Read the model definition and answer for the solid it produces. Units are mm, in the model's axes. A direction names the side the tool comes from. Coordinates: 2 decimals unless noted, no trailing zeros. Write each loop counter-clockwise with the first axis right and the second up, starting at its lowest first coordinate (ties: lowest second). Pieces come first, ordered by that corner, then holes.
(1) The mould has two halves that part along X. Classify faces 1 (the cylindrical face through (25.116, -3.788, 4.684)), 2 (the cylindrical face through (18.45, 9.9, 10.98)), 3 (the flat face through (-16, 9, 12.5)), 4 (the flat face through (-4.64, 5.73, 6.2)): +X half, -X half, draft (parallel to the pull), parting line (faces both ways), or undercut.
(2) Find the intervals of material crossed by probe 1 along X at (y, z) = (-18, 11.25); probe 2 along Z at (x, y) = (15.5, 17); probe 3 along Y at (x, z) = (12.5, 7.25), in increasing order.
(3) Section D-D on y = 21 is taken. Write down the section's boundary in (x, z), then the cut area to 3 significant figures.
(4) Section C-C on x = 11 is taken. Write down the section's boundary in (y, z).
(5) Section B-B on z = 1.5 is taken. Write down the section's boundary in (x, y).
(6) Section A-A on z = 7.75 is taken. Write down the section's boundary in (x, y), then the cut area to 3 significant figures.
(7) Given pin 1 (5 mm diameter, centred on y = 14, z = 5.5, fed in from +X); pin 2 (2 mm diameter, centred on y = 18.5, z = 5.5, fed in from -X); pin 3 (5 mm diameter, centred on x = 0.5, z = 5, fed in from -Y), each flat-ended and moving along its own axis, determine where each tip first touches the part or whether it passes through.
(8) Which of the six approach directions +Z, -Z, +X, -X, +Y, -Y give full straight-line access (tool end or side, diameter ignored) to faces 5 (the cylindrical face through (-0.3, -25.4, 4.7)), 6 (the flat face through (-5.75, 16, 6)), 7 (the cylindrical face through (-18.586, 9.132, 10.979)), 8 (the flat face through (11.19, -13.1, 6.2)), 9 (the cylindrical face through (20.037, 15.61, 4.684))?
from build123d import *

# Parameters (mm, degrees)
F0_R     = 3
F1_DEPTH = 3
F2_DEPTH = 9.5
F3_DEPTH = 12.5


with BuildPart() as f1:
    # F0 (on Top) → F1 (new body)
    with BuildSketch(Plane.XY):
        with BuildLine():
            ThreePointArc((3.552816, 4), (4.633236, 2.675), (5.24051, 1.076829))
            Line((5.24051, 1.076829), (9.370191, 1.229646))
            Line((9.370191, 1.229646), (24.300992, -7.390656))
            ThreePointArc((24.300992, -7.390656), (25.123746, -3.735961), (25.4, 0))
            ThreePointArc((25.4, 0), (19.889822, 15.79731), (5.75, 24.740604))
            Line((5.75, 24.740604), (5.75, 7.5))
            Line((5.75, 7.5), (3.552816, 4))
        make_face()
        with Locations((15.588457, 9)):
            Circle(F0_R, mode=Mode.SUBTRACT)
        with Locations((15.588457, 9)):
            Circle(F0_R)
        with BuildLine():
            ThreePointArc((-3.552816, 4), (0, 5.35), (3.552816, 4))
            Line((3.552816, 4), (5.75, 7.5))
            Line((5.75, 7.5), (5.75, 24.740604))
            ThreePointArc((5.75, 24.740604), (2.893843, 25.234613), (0, 25.4))
            ThreePointArc((0, 25.4), (-2.893843, 25.234613), (-5.75, 24.740604))
            Line((-5.75, 24.740604), (-5.75, 7.5))
            Line((-5.75, 7.5), (-3.552816, 4))
        make_face()
        with BuildLine():
            ThreePointArc((-5.24051, 1.076829), (-4.633236, 2.675), (-3.552816, 4))
            Line((-3.552816, 4), (-5.75, 7.5))
            Line((-5.75, 7.5), (-5.75, 24.740604))
            ThreePointArc((-5.75, 24.740604), (-21.997045, 12.7), (-24.300992, -7.390656))
            Line((-24.300992, -7.390656), (-9.370191, 1.229646))
            Line((-9.370191, 1.229646), (-5.24051, 1.076829))
        make_face()
        with Locations((-15.588457, 9)):
            Circle(F0_R, mode=Mode.SUBTRACT)
        with Locations((-15.588457, 9)):
            Circle(F0_R)
        with BuildLine():
            Line((-3.620191, -8.729646), (-1.687694, -5.076829))
            ThreePointArc((-1.687694, -5.076829), (-4.633236, -2.675), (-5.24051, 1.076829))
            Line((-5.24051, 1.076829), (-9.370191, 1.229646))
            Line((-9.370191, 1.229646), (-24.300992, -7.390656))
            ThreePointArc((-24.300992, -7.390656), (-23.300737, -10.111165), (-21.997045, -12.7))
            ThreePointArc((-21.997045, -12.7), (-20.406894, -15.123448), (-18.550992, -17.349948))
            Line((-18.550992, -17.349948), (-3.620191, -8.729646))
        make_face()
        with BuildLine():
            ThreePointArc((1.687694, -5.076829), (4.338874, -3.129963), (5.35, 0))
            ThreePointArc((5.35, 0), (5.322557, 0.54119), (5.24051, 1.076829))
            ThreePointArc((5.24051, 1.076829), (4.633236, 2.675), (3.552816, 4))
            ThreePointArc((3.552816, 4), (0, 5.35), (-3.552816, 4))
            ThreePointArc((-3.552816, 4), (-4.633236, 2.675), (-5.24051, 1.076829))
            ThreePointArc((-5.24051, 1.076829), (-4.633236, -2.675), (-1.687694, -5.076829))
            ThreePointArc((-1.687694, -5.076829), (0, -5.35), (1.687694, -5.076829))
        make_face()
        with BuildLine():
            ThreePointArc((5.24051, 1.076829), (5.322557, 0.54119), (5.35, 0))
            ThreePointArc((5.35, 0), (4.338874, -3.129963), (1.687694, -5.076829))
            Line((1.687694, -5.076829), (3.620191, -8.729646))
            Line((3.620191, -8.729646), (18.550992, -17.349948))
            ThreePointArc((18.550992, -17.349948), (20.406894, -15.123448), (21.997045, -12.7))
            ThreePointArc((21.997045, -12.7), (23.300737, -10.111165), (24.300992, -7.390656))
            Line((24.300992, -7.390656), (9.370191, 1.229646))
            Line((9.370191, 1.229646), (5.24051, 1.076829))
        make_face()
        with BuildLine():
            Line((3.620191, -8.729646), (1.687694, -5.076829))
            ThreePointArc((1.687694, -5.076829), (0, -5.35), (-1.687694, -5.076829))
            Line((-1.687694, -5.076829), (-3.620191, -8.729646))
            Line((-3.620191, -8.729646), (-18.550992, -17.349948))
            ThreePointArc((-18.550992, -17.349948), (0, -25.4), (18.550992, -17.349948))
            Line((18.550992, -17.349948), (3.620191, -8.729646))
        make_face()
        with Locations((0, -18)):
            Circle(F0_R, mode=Mode.SUBTRACT)
        with Locations((0, -18)):
            Circle(F0_R)
    extrude(amount=F1_DEPTH)

    # F0 (on Top) → F2 (join)
    with BuildSketch(Plane.XY):
        with BuildLine():
            ThreePointArc((-5.24051, 1.076829), (-4.633236, 2.675), (-3.552816, 4))
            Line((-3.552816, 4), (-5.75, 7.5))
            Line((-5.75, 7.5), (-5.75, 24.740604))
            ThreePointArc((-5.75, 24.740604), (-21.997045, 12.7), (-24.300992, -7.390656))
            Line((-24.300992, -7.390656), (-9.370191, 1.229646))
            Line((-9.370191, 1.229646), (-5.24051, 1.076829))
        make_face()
        with Locations((-15.588457, 9)):
            Circle(F0_R, mode=Mode.SUBTRACT)
        with Locations((-15.588457, 9)):
            Circle(F0_R)
        with Locations((15.588457, 9)):
            Circle(F0_R)
        with BuildLine():
            ThreePointArc((3.552816, 4), (4.633236, 2.675), (5.24051, 1.076829))
            Line((5.24051, 1.076829), (9.370191, 1.229646))
            Line((9.370191, 1.229646), (24.300992, -7.390656))
            ThreePointArc((24.300992, -7.390656), (25.123746, -3.735961), (25.4, 0))
            ThreePointArc((25.4, 0), (19.889822, 15.79731), (5.75, 24.740604))
            Line((5.75, 24.740604), (5.75, 7.5))
            Line((5.75, 7.5), (3.552816, 4))
        make_face()
        with Locations((15.588457, 9)):
            Circle(F0_R, mode=Mode.SUBTRACT)
        with BuildLine():
            Line((3.620191, -8.729646), (1.687694, -5.076829))
            ThreePointArc((1.687694, -5.076829), (0, -5.35), (-1.687694, -5.076829))
            Line((-1.687694, -5.076829), (-3.620191, -8.729646))
            Line((-3.620191, -8.729646), (-18.550992, -17.349948))
            ThreePointArc((-18.550992, -17.349948), (0, -25.4), (18.550992, -17.349948))
            Line((18.550992, -17.349948), (3.620191, -8.729646))
        make_face()
        with Locations((0, -18)):
            Circle(F0_R, mode=Mode.SUBTRACT)
        with Locations((0, -18)):
            Circle(F0_R)
    extrude(amount=F2_DEPTH)

    # F0 (on Top) → F3 (join)
    with BuildSketch(Plane.XY):
        with Locations((-15.588457, 9)):
            Circle(F0_R)
        with Locations((0, -18)):
            Circle(F0_R)
        with Locations((15.588457, 9)):
            Circle(F0_R)
    extrude(amount=F3_DEPTH)


solid = f1.part
Response:
1. face 1: +X half
1. face 2: undercut
1. face 3: draft
1. face 4: undercut
2. probe 1: x = -3 to 3
2. probe 2: z = 0 to 9.5
2. probe 3: y = -22.11 to -13.86, -0.58 to 22.11
3. outline: (-14.29, 0) - (14.29, 0) - (14.29, 9.5) - (5.75, 9.5) - (5.75, 3) - (-5.75, 3) - (-5.75, 9.5) - (-14.29, 9.5) - close
3. area: 197 mm2
4. outline: (-22.89, 0) - (22.89, 0) - (22.89, 9.5) - (0.29, 9.5) - (0.29, 3) - (-12.99, 3) - (-12.99, 9.5) - (-22.89, 9.5) - close
5. outline: (-24.3, -7.39) arc R25.4 ccw to (-22, -12.7) arc R25.4 ccw to (-18.55, -17.35) arc R25.4 ccw to (18.55, -17.35) arc R25.4 ccw to (22, -12.7) arc R25.4 ccw to (24.3, -7.39) arc R25.4 ccw to (25.4, 0) arc R25.4 ccw to (5.75, 24.74) arc R25.4 ccw to (0, 25.4) arc R25.4 ccw to (-5.75, 24.74) arc R25.4 ccw to start
6. outline: (-24.3, -7.39) - (-9.37, 1.23) - (-5.24, 1.08) arc R5.35 cw to (-3.55, 4) - (-5.75, 7.5) - (-5.75, 24.74) arc R25.4 ccw to start; (-18.55, -17.35) arc R25.4 ccw to (18.55, -17.35) - (3.62, -8.73) - (1.69, -5.08) arc R5.35 cw to (-1.69, -5.08) - (-3.62, -8.73) - close; (3.55, 4) arc R5.35 cw to (5.24, 1.08) - (9.37, 1.23) - (24.3, -7.39) arc R25.4 ccw to (25.4, 0) arc R25.4 ccw to (5.75, 24.74) - (5.75, 7.5) - close
6. area: 1,250 mm2
7. pin 1: stops at x = 22.65
7. pin 2: stops at x = -18.41
7. pin 3: stops at y = -25.4
8. face 5: +Z, -Z, -Y
8. face 6: +Z, +Y
8. face 7: +Z
8. face 8: +Z, +X
8. face 9: +Z, -Z, +X, +Y
